```python
from build123d import *

# Parameters (mm, degrees)
SKETCH1_R           = 17.5
SKETCH1_R_2         = 1.6
BOSS_EXTRUDE1_DEPTH = 10
SKETCH2_R           = 18.5
CUT_EXTRUDE1_DEPTH  = 4
SKETCH3_R           = 1.6
CUT_EXTRUDE2_DEPTH  = 224.991888552
SKETCH4_R           = 14
CUT_EXTRUDE3_DEPTH  = 224.991888552
SKETCH4_3_R         = 15.0625
SKETCH4_3_R_2       = 14
CUT_EXTRUDE4_DEPTH  = 7
FILLET1_R           = 4


with BuildPart() as part:
    # Sketch1 → Boss-Extrude1 (new body)
    with BuildSketch(Plane.XY.offset(37)):
        with BuildLine():
            Line((-25.534872354, -37.053613776), (126.113577761, -141.559582877))
            ThreePointArc((126.113577761, -141.559582877), (162.784444163, -136.592367058), (161.308367688, -99.616065541))
            Line((161.308367688, -99.616065541), (32.056602073, 31.581232775))
            ThreePointArc((32.056602073, 31.581232775), (-34.47199994, 28.925442436), (-25.534872354, -37.053613776))
        make_face()
        with Locations((141.718221977, -118.915707792)):
            Circle(SKETCH1_R, mode=Mode.SUBTRACT)
        with Locations((70.859110989, -59.457853896)):
            Circle(SKETCH1_R_2, mode=Mode.SUBTRACT)
        with Locations((93.840444282, -78.741482187)):
            Circle(SKETCH1_R_2, mode=Mode.SUBTRACT)
        with Locations((47.877777695, -40.174225605)):
            Circle(SKETCH1_R_2, mode=Mode.SUBTRACT)
        with Locations((47.767990244, 4.946625931)):
            Circle(SKETCH1_R_2, mode=Mode.SUBTRACT)
        with Locations((3.423348889, -47.901259716)):
            Circle(SKETCH1_R_2, mode=Mode.SUBTRACT)
        with Locations((68.973861607, -16.273907044)):
            Circle(SKETCH1_R_2, mode=Mode.SUBTRACT)
        with Locations((90.17973297, -37.494440018)):
            Circle(SKETCH1_R_2, mode=Mode.SUBTRACT)
        with Locations((28.003855203, -65.100059364)):
            Circle(SKETCH1_R_2, mode=Mode.SUBTRACT)
        with Locations((52.584361518, -82.298859012)):
            Circle(SKETCH1_R_2, mode=Mode.SUBTRACT)
    extrude(amount=BOSS_EXTRUDE1_DEPTH)

    # Sketch2 → Cut-Extrude1 (cut)
    with BuildSketch(Plane(origin=(0, 0, 37), x_dir=(-1, 0, 0), z_dir=(0, 0, -1))):
        with Locations((-141.718221977, -118.915707792)):
            Circle(SKETCH2_R)
    extrude(amount=-CUT_EXTRUDE1_DEPTH, mode=Mode.SUBTRACT)

    # Sketch3 → Cut-Extrude2 (cut, through all)
    with BuildSketch(Plane(origin=(0, 0, 37), x_dir=(-1, 0, 0), z_dir=(0, 0, -1))):
        with Locations((-18.75, 32.475952642)):
            Circle(SKETCH3_R)
        with Locations((6.511806663, 36.930290738)):
            Circle(SKETCH3_R)
        with Locations((28.726666617, 24.104535363)):
            Circle(SKETCH3_R)
        with Locations((37.5, 0)):
            Circle(SKETCH3_R)
        with Locations((28.726666617, -24.104535363)):
            Circle(SKETCH3_R)
    extrude(amount=-CUT_EXTRUDE2_DEPTH, mode=Mode.SUBTRACT)

    # Sketch4 → Cut-Extrude3 (cut, through all)
    with BuildSketch(Plane(origin=(0, 0, 37), x_dir=(-1, 0, 0), z_dir=(0, 0, -1))):
        Circle(SKETCH4_R)
    extrude(amount=-CUT_EXTRUDE3_DEPTH, mode=Mode.SUBTRACT)

    # Sketch4<3> → Cut-Extrude4 (cut)
    with BuildSketch(Plane(origin=(0, 0, 37), x_dir=(-1, 0, 0), z_dir=(0, 0, -1))):
        Circle(SKETCH4_3_R)
        Circle(SKETCH4_3_R_2, mode=Mode.SUBTRACT)
    extrude(amount=-CUT_EXTRUDE4_DEPTH, mode=Mode.SUBTRACT)

    # Fillet1
    fillet1_edges = [part.edges().sort_by_distance(p)[0] for p in [
        (162.784444163, -136.592367058, 47),
        (96.68248488, -34.017416383, 47),
        (-34.47199994, 28.925442436, 47),
        (50.289352703, -89.306598327, 47),
    ]]
    fillet(fillet1_edges, radius=FILLET1_R)


solid = part.part
```
Build history of the part. All positions in model axes, mm. A direction names the side the tool comes from. Round coordinates to 2 decimals unless told otherwise and drop trailing zeros. Use a Markdown table: item, result.
1) Wall check: L1, parallel to X at y = 1, z = 41; L2, parallel to X at y = 1, z = 45.5; L3, parallel to Y at x = 130.5, z = 44. Give the ranges that are in metal, low to high.
Recorded:
| item | result |
|---|---|
| L1 | x = -44.99 to -38.75, -36.25 to -15.03, 15.03 to 62.18 |
| L2 | x = -44.11 to -38.75, -36.25 to -13.96, 13.96 to 60.95 |
| L3 | y = -143.88 to -132.35, -105.48 to -68.52 |
2) Tool access for faces 1 (the face through (153, -133, 41)), 2 (the face through (-33.79, 29.72, 39.96)): list every direction of +Z, -Z, +X, -X, +Y, -Y with a clear straight run to the whole face (end or side of a thin tool).
Recorded:
| item | result |
|---|---|
| face 1 | -Z |
| face 2 | +Z, -Z |
3) Pull direction Y, two halves, no side cores. Call faces 3 (the face through (11.95, -9.17, 40.45)), 4 (the face through (124.235, -118.146, 43.958)), 5 (the face through (94.965, -33.9, 45.797)), 6 (the face through (54, -50, 47)): pulls with the +Y half, pulls with the -Y half, needs draft (parallel to the pull), parting line crosses it, or undercut.
Recorded:
| item | result |
|---|---|
| face 3 | undercut |
| face 4 | undercut |
| face 5 | pulls with the +Y half |
| face 6 | needs draft |
4) Flat gauge pins, fed straight in: pin 1 Ø4 at (y, z) = (-12, 44) entering from +X; pin 2 Ø1.5 at (x, z) = (35, 41.5) entering from +Y; pin 3 Ø1.5 at (y, z) = (24, 38.5) entering from -X. Where does each tip first touch, or does it go through?
Recorded:
| item | result |
|---|---|
| pin 1 | stops at x = 76.86 |
| pin 2 | stops at y = 29.35 |
| pin 3 | stops at x = -38.53 |
5) Saw through at A-A on z = 39.25. Give the number of separate pieces and of enclosed holes in the cut face, and give its area (3 significant figures).
Recorded:
| item | result |
|---|---|
| separate pieces | 1 |
| enclosed holes | 16 |
| area | 15,900 mm² |
